Geometry: final body of the model. Coordinates: model frame, mm. Coordinates: 2 decimals unless noted, no trailing zeros. Loops run counter-clockwise (first coordinate to the right, second up) from the corner with the lowest first, then second, coordinate; pieces in that order, holes last. Notation, with made-up numbers: (24.5, 61) - (30.5, 61) arc R27 cw to (30.5, 85) - close; hole circle Ø2 at (13, 77.5). An arc over 180 degrees is marked (long way). Answer in a Markdown table with one row per item.
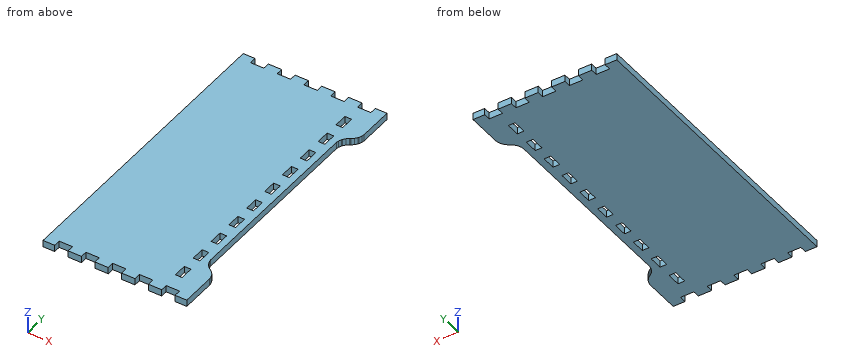
from build123d import *

# Parameters (mm, degrees)
BOSS_EXTRUDE1_DEPTH = 5.715


with BuildPart() as part:
    # Model → Boss-Extrude1 (new body)
    with BuildSketch(Plane.XY):
        Polygon((1156.43152, 23.2006394), (1166.42388, 23.2006394), (1166.42388, 28.91536), (1177.85388, 28.91536), (1177.85388, 23.2006394), (1189.28388, 23.2006394), (1189.28388, 28.91536), (1200.71388, 28.91536), (1200.71388, 23.2006394), (1212.14388, 23.2006394), (1212.14388, 28.91536), (1223.57388, 28.91536), (1223.57388, 23.2006394), (1235.00388, 23.2006394), (1235.00388, 28.91536), (1246.43388, 28.91536), (1246.43388, 23.2006394), (1257.86388, 23.2006394), (1257.86388, 28.91536), (1269.29388, 28.91536), (1269.29388, 23.2006394), (1279.28878, 23.2006394), (1279.28878, 51.775868), (1279.28878, 52.515516), (1278.90016, 54.734206), (1278.00862, 57.056274), (1277.75716, 57.49036), (1277.50824, 57.925716), (1275.94106, 59.857894), (1274.00812, 61.423296), (1273.57378, 61.673994), (1273.13944, 61.924946), (1271.2065, 63.491872), (1269.63932, 65.423796), (1269.3904, 65.857882), (1269.13894, 66.293238), (1268.24994, 68.615306), (1267.85878, 70.833996), (1267.85878, 71.572628), (1267.85878, 231.25811), (1267.85878, 231.998266), (1268.24994, 234.216956), (1269.13894, 236.539024), (1269.3904, 236.972856), (1269.63932, 237.408466), (1271.2065, 239.34039), (1273.13944, 240.906046), (1273.57378, 241.156744), (1274.00812, 241.407696), (1275.94106, 242.974368), (1277.50824, 244.906546), (1277.75716, 245.340378), (1278.00862, 245.775988), (1278.90016, 248.098056), (1279.28878, 250.316746), (1279.28878, 251.055124), (1279.28878, 279.63114), (1269.29388, 279.63114), (1269.29388, 273.91614), (1257.86388, 273.91614), (1257.86388, 279.63114), (1246.43388, 279.63114), (1246.43388, 273.91614), (1235.00388, 273.91614), (1235.00388, 279.63114), (1223.57388, 279.63114), (1223.57388, 273.91614), (1212.14388, 273.91614), (1212.14388, 279.63114), (1200.71388, 279.63114), (1200.71388, 273.91614), (1189.28388, 273.91614), (1189.28388, 279.63114), (1177.85388, 279.63114), (1177.85388, 273.91614), (1166.42388, 273.91614), (1166.42388, 279.63114), (1156.43152, 279.63114), align=None)
        Polygon((1262.14378, 48.545496), (1262.14378, 42.83075), (1256.43132, 42.83075), (1256.43132, 54.260496), (1262.14378, 54.260496), align=None, mode=Mode.SUBTRACT)
        Polygon((1262.14378, 71.40575), (1262.14378, 65.691004), (1256.43132, 65.691004), (1256.43132, 77.120496), (1262.14378, 77.120496), align=None, mode=Mode.SUBTRACT)
        Polygon((1262.14378, 94.266004), (1262.14378, 88.549988), (1256.43132, 88.549988), (1256.43132, 99.98075), (1262.14378, 99.98075), align=None, mode=Mode.SUBTRACT)
        Polygon((1262.14378, 117.124988), (1262.14378, 111.410496), (1256.43132, 111.410496), (1256.43132, 122.841004), (1262.14378, 122.841004), align=None, mode=Mode.SUBTRACT)
        Polygon((1262.14378, 139.985496), (1262.14378, 134.270496), (1256.43132, 134.270496), (1256.43132, 145.699988), (1262.14378, 145.699988), align=None, mode=Mode.SUBTRACT)
        Polygon((1262.14378, 162.845496), (1262.14378, 157.13075), (1256.43132, 157.13075), (1256.43132, 168.560496), (1262.14378, 168.560496), align=None, mode=Mode.SUBTRACT)
        Polygon((1262.14378, 185.70575), (1262.14378, 179.991004), (1256.43132, 179.991004), (1256.43132, 191.420496), (1262.14378, 191.420496), align=None, mode=Mode.SUBTRACT)
        Polygon((1262.14378, 208.566004), (1262.14378, 202.849988), (1256.43132, 202.849988), (1256.43132, 214.28075), (1262.14378, 214.28075), align=None, mode=Mode.SUBTRACT)
        Polygon((1262.14378, 231.424988), (1262.14378, 225.710496), (1256.43132, 225.710496), (1256.43132, 237.141004), (1262.14378, 237.141004), align=None, mode=Mode.SUBTRACT)
        Polygon((1262.14378, 254.28448), (1262.14378, 248.570496), (1256.43132, 248.570496), (1256.43132, 259.99948), (1262.14378, 259.99948), align=None, mode=Mode.SUBTRACT)
    extrude(amount=BOSS_EXTRUDE1_DEPTH)


solid = part.part
(1) First-contact query: pin 1 Ø1.7 at (y, z) = (208.5, 2) entering from +X; pin 2 Ø1.7 at (x, z) = (1260.5, 3) entering from -Y; pin 3 Ø3 at (x, z) = (1260, 2.5) entering from +Y. Flat tips, straight axial feed; report the tip coordinate or a pass-through.
Verdict:
| item | result |
|---|---|
| pin 1 | stops at x = 1267.86 |
| pin 2 | stops at y = 28.92 |
| pin 3 | stops at y = 273.92 |
(2) Cut plane B-B on x = 1175. Output: boundary loops of the cut face in (y, z) (3 decimals).
Verdict:
| item | result |
|---|---|
| outline | (28.915, 0) - (273.916, 0) - (273.916, 5.715) - (28.915, 5.715) - close |
(3) Cut plane C-C on y = 255.5. Output: boundary loops of the cut face in (x, z) (3 decimals).
Verdict:
| item | result |
|---|---|
| outline | (1156.432, 0) - (1256.431, 0) - (1256.431, 5.715) - (1156.432, 5.715) - close; (1262.144, 0) - (1279.289, 0) - (1279.289, 5.715) - (1262.144, 5.715) - close |
(4) Ray query, probe 1 along X at (y, z) = (160.5, 2.25); probe 2 along X at (y, z) = (50.5, 1.65); probe 3 along X at (y, z) = (129, 4.8). Return the intervals inside material, ascending.
Verdict:
| item | result |
|---|---|
| probe 1 | x = 1156.43 to 1256.43, 1262.14 to 1267.86 |
| probe 2 | x = 1156.43 to 1256.43, 1262.14 to 1279.29 |
| probe 3 | x = 1156.43 to 1267.86 |
(5) Cut plane D-D on z = 1.2. State how many separate pieces and enclosed holes the cut face has, then the cut area to 3 significant figures.
Verdict:
| item | result |
|---|---|
| separate pieces | 1 |
| enclosed holes | 10 |
| area | 28,100 mm² |
(6) Cut plane A-A on y = 118. Output: boundary loops of the cut face in (x, z) (3 decimals).
Verdict:
| item | result |
|---|---|
| outline | (1156.432, 0) - (1256.431, 0) - (1256.431, 5.715) - (1156.432, 5.715) - close; (1262.144, 0) - (1267.859, 0) - (1267.859, 5.715) - (1262.144, 5.715) - close |
